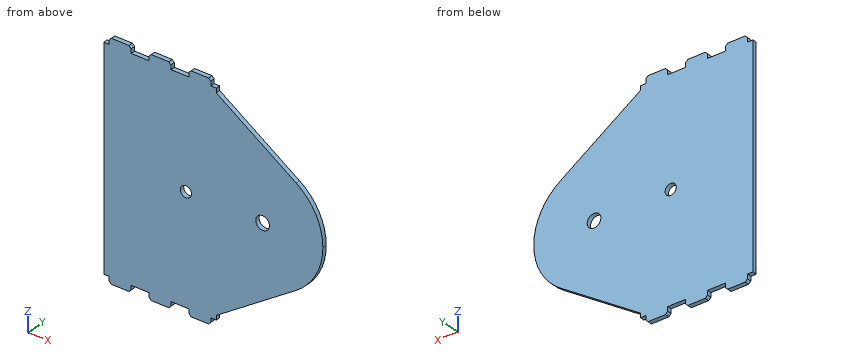
from build123d import *

# Parameters (mm, degrees)
SM_BASE_FLANGE_1_DEPTH = 4
OTHER_1_DEPTH          = 4


# Read off the part's stored shape, not the designer's step: Выступы и прорези-Выступ1
# Sheet-metal steps are written as plain solids
with BuildPart() as part:
    # Sketch 1 → Базовая кромка1 (new body)
    with BuildSketch(Plane(origin=(0, 0, 0), x_dir=(1, 0, 0), z_dir=(0, 1, 0))):
        with BuildLine():
            Line((-145, -98.667725183), (-145, 0))
            Line((-145, 0), (-75.1, 0))
            ThreePointArc((-75.1, 0), (-70, -5.1), (-64.9, 0))
            Line((-64.9, 0), (-6.25, 0))
            ThreePointArc((-6.25, 0), (0, -6.25), (6.25, 0))
            Line((6.25, 0), (55, 0))
            ThreePointArc((55, 0), (48.538654235, -25.865015853), (30.672761998, -45.652838591))
            Line((30.672761998, -45.652838591), (-42.280195622, -94.667725183))
            Line((-42.280195622, -94.667725183), (-42.280195622, -98.667725183))
            Line((-42.280195622, -98.667725183), (-145, -98.667725183))
        make_face()
    extrude(amount=SM_BASE_FLANGE_1_DEPTH)

    # Other 1 outline → Other 1 (add)
    with BuildSketch(Plane(origin=(0, 0, 0), x_dir=(1, 0, 0), z_dir=(0, 1, 0))):
        Polygon((-47.280195622, -98.667725183), (-67.280195622, -98.667725183), (-67.280195622, -102.667725183), (-65.280195622, -104.667725183), (-49.280195622, -104.667725183), (-47.280195622, -102.667725183), align=None)
        Polygon((-83.640097811, -98.667725183), (-103.640097811, -98.667725183), (-103.640097811, -102.667725183), (-101.640097811, -104.667725183), (-85.640097811, -104.667725183), (-83.640097811, -102.667725183), align=None)
        Polygon((-140, -98.667725183), (-140, -102.667725183), (-138, -104.667725183), (-122, -104.667725183), (-120, -102.667725183), (-120, -98.667725183), align=None)
    extrude(amount=OTHER_1_DEPTH)

    # Зеркальное отражение1: part across plane


with BuildPart() as part_1:
    add(part.part)
    add(part.part.mirror(Plane(origin=(-145, 4, 0), x_dir=(1, 0, 0), z_dir=(0, 0, 1))))


solid = part_1.part
The listing builds one solid part. Answer for the finished solid, in the listing's coordinates (mm). Give positions to 0.01 mm unless a question says otherwise; leave off trailing zeros. Order: outer loops, then holes, each group sorted by start corner. A loop starts at its lowest first (then second) coordinate and runs counter-clockwise, first axis right, second up. Notation, with made-up numbers: (75, 16.25) - (94, 16.25) arc R13 ccw to (94, 21.25) - close; hole circle Ø8 at (-7, -36.5). An arc over 180 degrees is marked (long way). Use one line per item in the form item = value.
1) Find section C-C on z = 37.5. Determine the outline of the cut face in (x, y), and give its area (3 significant figures).
Verdict:
outline = (-145, 0) - (40.23, 0) - (40.23, 4) - (-145, 4) - close
area = 741 mm^2
2) Consider probe 1 along Z at (x, y) = (-70, 1.85); probe 2 along Z at (x, y) = (0, 2.8); probe 3 along Z at (x, y) = (-109.5, 1.7). Determine where each line is inside the solid, lowest interval first. Write a range as [from, to].
Verdict:
probe_1 = [-98.67, -5.1], [5.1, 98.67]
probe_2 = [-66.26, -6.25], [6.25, 66.26]
probe_3 = [-98.67, 98.67]
3) Find section D-D on x = 0. Determine the outline of the cut face in (y, z), and give its area (3 significant figures).
Verdict:
outline = (0, -66.26) - (4, -66.26) - (4, -6.25) - (0, -6.25) - close; (0, 6.25) - (4, 6.25) - (4, 66.26) - (0, 66.26) - close
area = 480 mm^2
4) Each of these flat-tipped pins is pushed along its axis until it touches: pin 1 (3 mm diameter, centred on x = -94, z = -11, fed in from -Y); pin 2 (1.2 mm diameter, centred on y = 1.5, z = -100.5, fed in from -X); pin 3 (2 mm diameter, centred on x = -109, y = 2, fed in from -Z). Where does it stop, or does it pass through?
Verdict:
pin_1 = 0
pin_2 = -140
pin_3 = -98.67
5) Find section A-A on x = -70. Determine the outline of the cut face in (y, z).
Verdict:
outline = (0, -98.67) - (4, -98.67) - (4, -5.1) - (0, -5.1) - close; (0, 5.1) - (4, 5.1) - (4, 98.67) - (0, 98.67) - close
6) Find section B-B on y = 3.4. Give the number of separate pieces and of enclosed holes in the cut face, and give its area (3 significant figures).
Verdict:
separate_pieces = 1
enclosed_holes = 2
area = 32,600 mm^2
